Can you work these out from the model? Positions are in its coordinate system, mm. Give positions to 0.01 mm unless a question says otherwise; leave off trailing zeros. Loops run counter-clockwise (first coordinate to the right, second up) from the corner with the lowest first, then second, coordinate; pieces in that order, holes last. Notation, with made-up numbers: M 15.25,-23 L 57.25,-23 A20 cw 57.25,-3 Z; hole C -18.75,58.25 d1. An arc over 180 degrees is marked long. Use CSV: the item, a comma, the result in double quotes.
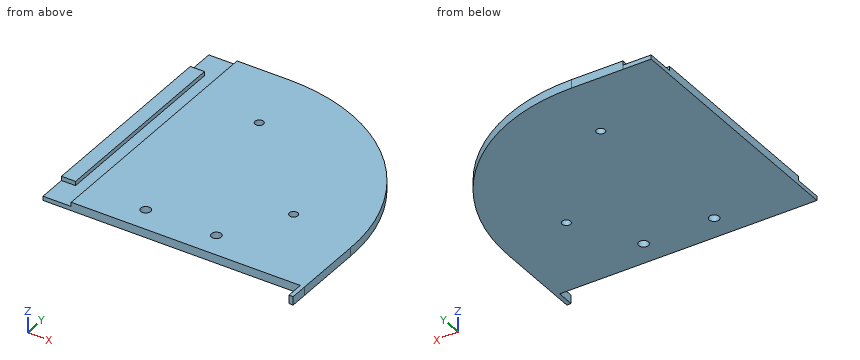
Solid Edge part; units mm, degrees
sketch "Sketch1" plane through (0, 0, 0) normal (0, 0, 1) x (1, 0, 0)
  line L0 (0, 0) -> (0, 180.07)
  line L1 (0, 180.07) -> (36.535, 180.07)
  arc A0 (36.535, 180.07) -> (165.365, 50) centre (36.535, 51.2341) cw
  line L2 (165.365, 0) -> (165.365, 50)
  line L3 (0, 0) -> (165.365, 0)
  circle A1 centre (47.06, 132.1) radius 2.9988
  circle A2 centre (117.55, 61.39) radius 2.9988
  dimension "D1" = 165.365
extrude "Protrusion1" add sketch "Sketch1" along normal blind 6
sketch "Sketch2" plane through (0, 90.035, 3) normal (-1, 0, 0) x (0, -1, 0)
  line L0 (-90.035, 3) -> (90.035, 3)
  line L1 (90.035, 3) -> (90.035, -3)
  line L2 (90.035, -3) -> (-90.035, -3)
  line L3 (-90.035, -3) -> (-90.035, 3)
extrude "Extrusionsausprägung_2" add sketch "Sketch2" along normal blind 20
sketch "Sketch3" plane through (72.6855, 90.035, 6) normal (0, 0, 1) x (1, 0, 0)
  line L0 (-92.6855, -70) -> (-82.6855, -70)
  line L1 (-82.6855, -70) -> (-82.6855, 70)
  line L2 (-82.6855, 70) -> (-92.6855, 70)
  line L3 (-92.6855, 70) -> (-92.6855, 90.035)
  line L4 (-92.6855, 90.035) -> (-72.6855, 90.035)
  line L5 (-72.6855, 90.035) -> (-72.6855, -90.035)
  line L6 (-72.6855, -90.035) -> (-92.6855, -90.035)
  line L7 (-92.6855, -90.035) -> (-92.6855, -70)
  dimension "D1" = 82.6855
extrude "Extrusionsausschnitt_1" cut sketch "Sketch3" against normal blind 3
sketch "Sketch4" plane through (72.6855, 90.035, 0) normal (0, 0, -1) x (0, 1, 0)
  circle A0 centre (-72.515, -31.2255) radius 3.5
  circle A1 centre (-72.515, 18.7745) radius 3.5
  dimension "D1" = 72.515
extrude "Cutout1" cut sketch "Sketch4" against normal through all
sketch "Sketch5" plane through (72.6825, 0, 3) normal (0, -1, 0) x (-1, 0, 0)
  line L0 (-92.6825, 3) -> (-89.6825, 3)
  line L1 (-89.6825, 3) -> (-89.6825, -3)
  line L2 (-89.6825, -3) -> (-92.6825, -3)
  line L3 (-92.6825, -3) -> (-92.6825, 3)
extrude "Extrusionsausprägung_3" add sketch "Sketch5" along normal blind 12.4
properties material "Nylon, allgemein"
Q1. I want a section at A-A, the plane z = 3.95. Please give me the cut outline in (x, y) (3 decimals), then the cut area to 3 significant figures.
Model answer:
outline,"M -20,20.035 L -10,20.035 L -10,160.035 L -20,160.035 Z; M 0,0 L 162.365,0 L 162.365,-12.4 L 165.365,-12.4 L 165.365,0 L 165.365,50 A128.836 ccw 36.535,180.07 L 0,180.07 Z; hole C 41.46,17.52 d7; hole C 47.06,132.1 d5.998; hole C 91.46,17.52 d7; hole C 117.55,61.39 d5.998"
area,"27,500 mm2"
Q2. I want a section at C-C, the plane y = 132.1. Please give me the cut outline in (x, z).
Model answer:
outline,"M -20,0 L 44.06,0 L 44.06,6 L 0,6 L 0,3 L -10,3 L -10,6 L -20,6 Z; M 50.06,0 L 136.83,0 L 136.83,6 L 50.06,6 Z"
Q3. I'm going to push flat-ended pins straight in: P1, Ø1.5, axis at x = -15.5, z = 5, coming from the +Y side (3 decimals); P2, Ø4, axis at x = 88, y = 40.5, coming from the -Z side; P3, Ø1.5, axis at y = 108, z = 4.5, coming from the +X side; P4, Ø1.8, axis at y = -6.5, z = 3, coming from the -X side (3 decimals). Where does each tip first touch, or does it pass through?
Model answer:
P1,"y = 160.035"
P2,"z = 0"
P3,"x = 152.56"
P4,"x = 162.365"
Q4. I want a section at B-B, the plane x = 91.46. Please give me the cut outline in (y, z), then the cut area to 3 significant figures.
Model answer:
outline,"M 0,0 L 14.02,0 L 14.02,6 L 0,6 Z; M 21.02,0 L 167.78,0 L 167.78,6 L 21.02,6 Z"
area,"965 mm2"
Q5. Please list where these lines run through material, in increasing order: L1, parallel to X at y = 17.52, z = 2.8; L2, parallel to X at y = 17.52, z = 3.8; L3, parallel to X at y = 53.5, z = 3.3. Write a range as from..to.
Model answer:
L1,"-20..37.96, 44.96..87.96, 94.96..165.37"
L2,"0..37.96, 44.96..87.96, 94.96..165.37"
L3,"-20..-10, 0..165.35"
Q6. I want a section at D-D, the plane y = 157.5. Please give me the cut outline in (x, z), then the cut area to 3 significant figures.
Model answer:
outline,"M -20,0 L 109.38,0 L 109.38,6 L 0,6 L 0,3 L -10,3 L -10,6 L -20,6 Z"
area,"746 mm2"
